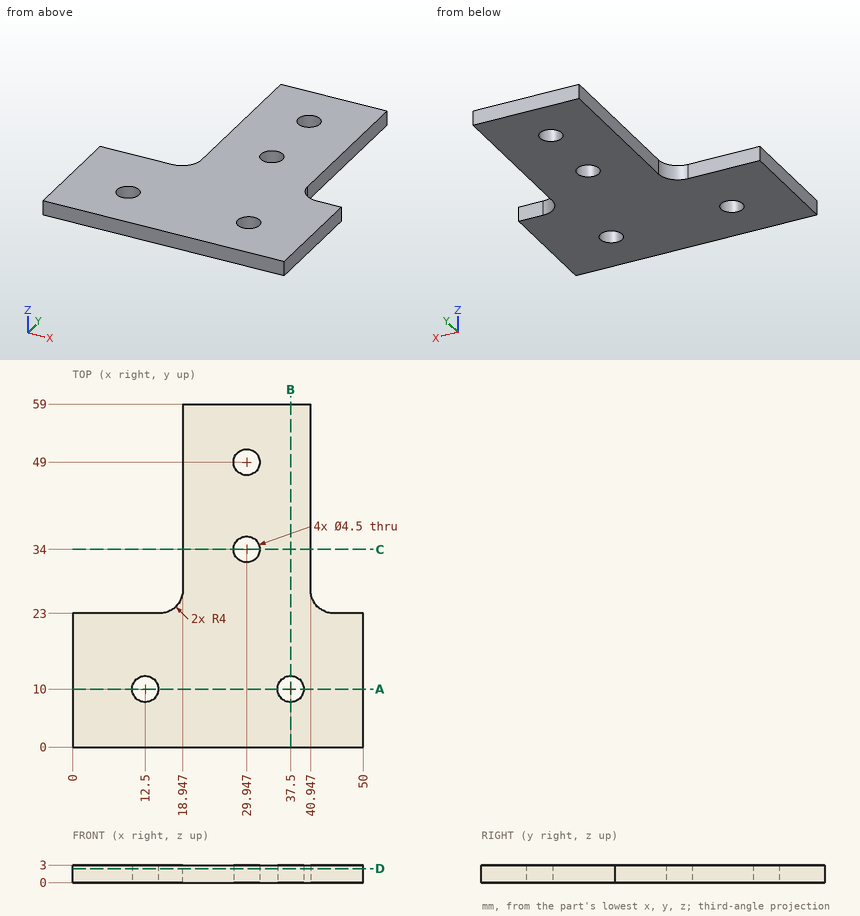
Geometry check sheet. Reference: drawing and pictorial views, mm from the part's lowest x, y, z. Give positions to 0.01 mm unless a question says otherwise; leave off trailing zeros. Order: outer loops, then holes, each group sorted by start corner. A loop starts at its lowest first (then second) coordinate and runs counter-clockwise, first axis right, second up. Notation, with made-up numbers: M 77.5,2.25 L 112.5,2.25 A21 ccw 112.5,16.25 Z; hole C 25.25,-5.75 d3. An arc over 180 degrees is marked long. Answer in a Markdown table with one row per item. Add a question column.
Item 1: Section check A-A, the plane y = 10. Enter the section's corners in (x, z), and give its area (3 significant figures).
Item 2: Section check C-C, the plane y = 34. Enter the section's corners in (x, z), and give its area (3 significant figures).
Item 3: Scan lines: probe 1 along Y at (x, z) = (12.5, 2.35); probe 2 along Y at (x, z) = (37.5, 1.65); probe 3 along X at (y, z) = (54, 1.7). Record each from-to range of solid material in increasing order. Write a range as from..to.
Item 4: Gauge pin test, flat ends, axial feed: pin 1 (1.5 mm diameter, centred on x = 8.5, z = 1, fed in from +Y); pin 2 (10 mm diameter, centred on x = 25.5, y = 50, fed in from -Z); pin 3 (0.9 mm diameter, centred on y = 36.5, z = 2, fed in from -X). Record the tip position at first contact, or that the pin passes through.
Item 5: Section check B-B, the plane x = 37.5. Enter the section's corners in (y, z).
Item 6: Section check D-D, the plane z = 2.4. Enter the section's corners in (x, y), and give its area (3 significant figures).
Filled sheet:
| question | item | result |
|---|---|---|
| 1 | outline | M 0,0 L 10.25,0 L 10.25,3 L 0,3 Z; M 14.75,0 L 35.25,0 L 35.25,3 L 14.75,3 Z; M 39.75,0 L 50,0 L 50,3 L 39.75,3 Z |
| 1 | area | 123 mm^2 |
| 2 | outline | M 18.95,0 L 27.7,0 L 27.7,3 L 18.95,3 Z; M 32.2,0 L 40.95,0 L 40.95,3 L 32.2,3 Z |
| 2 | area | 52.5 mm^2 |
| 3 | probe 1 | y = 0..7.75, 12.25..23 |
| 3 | probe 2 | y = 0..7.75, 12.25..59 |
| 3 | probe 3 | x = 18.95..40.95 |
| 4 | pin 1 | stops at y = 23 |
| 4 | pin 2 | stops at z = 0 |
| 4 | pin 3 | stops at x = 18.95 |
| 5 | outline | M 0,0 L 7.75,0 L 7.75,3 L 0,3 Z; M 12.25,0 L 59,0 L 59,3 L 12.25,3 Z |
| 6 | outline | M 0,0 L 50,0 L 50,23 L 44.95,23 A4 cw 40.95,27 L 40.95,59 L 18.95,59 L 18.95,27 A4 cw 14.95,23 L 0,23 Z; hole C 12.5,10 d4.5; hole C 29.95,34 d4.5; hole C 29.95,49 d4.5; hole C 37.5,10 d4.5 |
| 6 | area | 1,890 mm^2 |
